```python
from build123d import *

# Parameters (mm, degrees)
SKETCH1_R           = 15
SKETCH1_R_2         = 4
SKETCH1_R_3         = 1.5
BOSS_EXTRUDE1_DEPTH = 1
SKETCH1_4_R         = 4
SKETCH1_4_R_2       = 3.2
BOSS_EXTRUDE2_DEPTH = 11
SKETCH1_5_R         = 3.2
BOSS_EXTRUDE3_DEPTH = 8
FILLET1_R           = 2


with BuildPart() as part:
    # Sketch1 → Boss-Extrude1 (new body)
    with BuildSketch(Plane.XY):
        Circle(SKETCH1_R)
        Circle(SKETCH1_R_2, mode=Mode.SUBTRACT)
        with Locations((0, 12.5)):
            Circle(SKETCH1_R_3, mode=Mode.SUBTRACT)
        with Locations((12.5, 0)):
            Circle(SKETCH1_R_3, mode=Mode.SUBTRACT)
        with Locations((0, -12.5)):
            Circle(SKETCH1_R_3, mode=Mode.SUBTRACT)
        with Locations((-12.5, 0)):
            Circle(SKETCH1_R_3, mode=Mode.SUBTRACT)
    extrude(amount=BOSS_EXTRUDE1_DEPTH)

    # Sketch1<4> → Boss-Extrude2 (add)
    with BuildSketch(Plane.XY):
        Circle(SKETCH1_4_R)
        Circle(SKETCH1_4_R_2, mode=Mode.SUBTRACT)
    extrude(amount=BOSS_EXTRUDE2_DEPTH)

    # Sketch1<5> → Boss-Extrude3 (add)
    with BuildSketch(Plane.XY):
        Circle(SKETCH1_5_R)
    extrude(amount=BOSS_EXTRUDE3_DEPTH)

    # Fillet1
    fillet1_edges = [part.edges().sort_by_distance(p)[0] for p in [
        (-4, 0, 1),
    ]]
    fillet(fillet1_edges, radius=FILLET1_R)


solid = part.part
```
Geometry check sheet. Reference: the model listing, model coordinates, mm. A direction names the side the tool comes from. Round coordinates to 2 decimals unless told otherwise and drop trailing zeros. Loops run counter-clockwise (first coordinate to the right, second up) from the corner with the lowest first, then second, coordinate; pieces in that order, holes last. Notation, with made-up numbers: M 87,51.5 L 146,51.5 A22 cw 146,60.5 Z; hole C -24,-2.75 d6. An arc over 180 degrees is marked long. Return JSON: item names as keys, results as strings. Group by question number.
(1) Section check C-C, the plane z = 10.25. Enter the section's corners in (x, y).
(2) Section check A-A, the plane x = -12.5. Enter the section's corners in (y, z), and give its area (3 significant figures).
(3) Section check B-B, the plane y = 0. Enter the section's corners in (x, z), and give its area (3 significant figures).
(4) Mould release check, pull along Y, two halves, no side actions. Record for faces 3 (the face through (-14.985, 0.66, 0.493)), 4 (the face through (-14, 0.07, 0.49)), 5 (the face through (0, 0, 0)): pulls with the +Y half, pulls with the -Y half, needs draft (parallel to the pull), parting line crosses it, or undercut.
(5) Go/stop test with flat-tipped pins: pin 1 (1.8 mm diameter, centred on x = 0, y = 12.5, fed in from -Z); pin 2 (4 mm diameter, centred on y = 6.5, z = 2.5, fed in from +X); pin 3 (8 mm diameter, centred on x = 8, y = -4.5, fed in from +Z); pin 4 (5 mm diameter, centred on x = -7.5, z = 2.5, fed in from +Y). Record where each tip stops, or that it passes through.
(6) Set-up check for faces 1 (the face through (11, 0.07, 0.49)), 2 (the face through (-0.867, -3.905, 6.944)): record each of +Z, -Z, +X, -X, +Y, -Y from which the full face is reachable in a straight line by a thin tool's end or side.
(7) Scan lines: line 1 along Y through (x, z) = (0, 0.3); line 2 along Z through (x, y) = (10, -1); line 3 along Y through (x, z) = (-1, 9.75). Record each from-to range of solid material in increasing order. Write a range as [from, to].
Data:
{
 "1": {"outline": "C 0,0 d8; hole C 0,0 d6.4"},
 "2": {"outline": "M -8.29,0 L -1.5,0 L -1.5,1 L -8.29,1 Z; M 1.5,0 L 8.29,0 L 8.29,1 L 1.5,1 Z", "area": "13.6 mm²"},
 "3": {"outline": "M -15,0 L -14,0 L -14,1 L -15,1 Z; M -11,0 L 11,0 L 11,1 L 6,1 A2 cw 4,3 L 4,11 L 3.2,11 L 3.2,8 L -3.2,8 L -3.2,11 L -4,11 L -4,3 A2 cw -6,1 L -11,1 Z; M 14,0 L 15,0 L 15,1 L 14,1 Z", "area": "86.5 mm²"},
 "4": {"face 3": "parting line crosses it", "face 4": "undercut", "face 5": "needs draft"},
 "5": {"pin 1": "through", "pin 2": "x = 14.08", "pin 3": "z = 1.18", "pin 4": "y = 13.96"},
 "6": {"face 1": "+Z, -Z", "face 2": "+Z"},
 "7": {"line 1": "[-15, -14], [-11, 11], [14, 15]", "line 2": "[0, 1]", "line 3": "[-3.87, -3.04], [3.04, 3.87]"}
}
